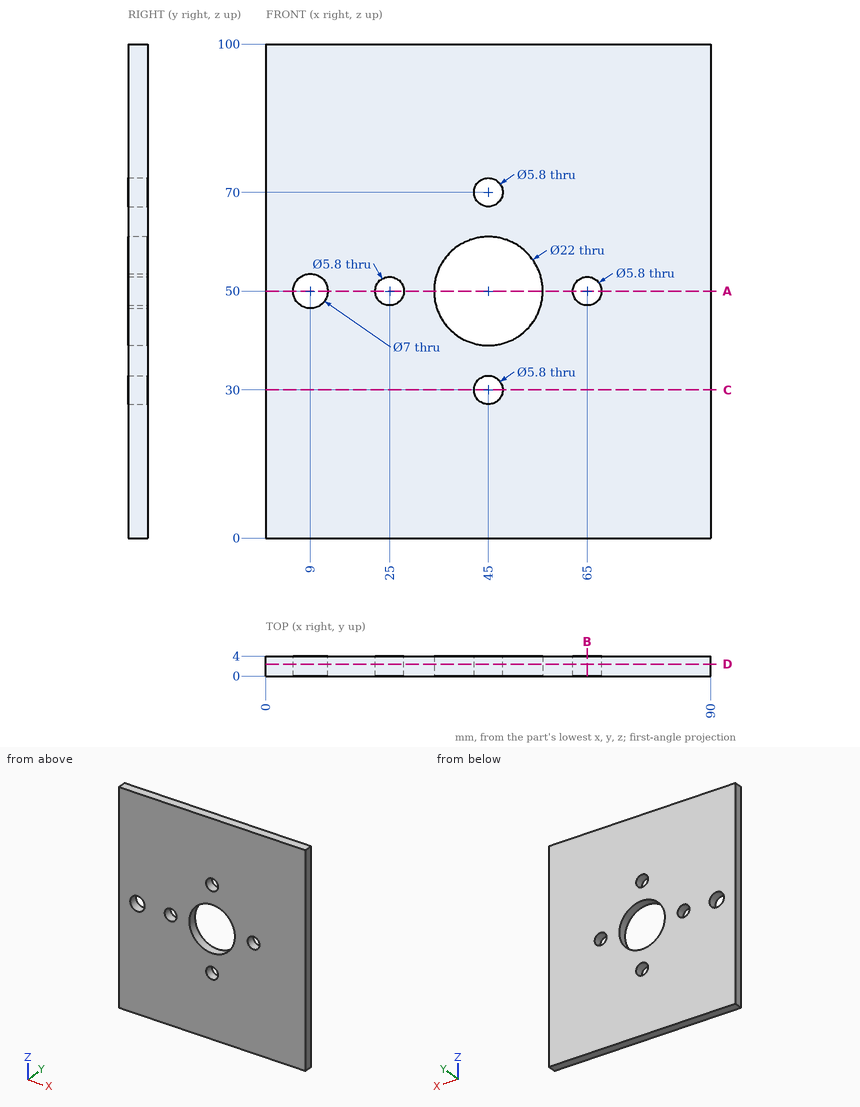
Check sheet for the drawn part. Datum: minimum x, y, z corner. Units: mm. Round coordinates to 2 decimals unless told otherwise and drop trailing zeros. Write each loop counter-clockwise with the first axis right and the second up, starting at its lowest first coordinate (ties: lowest second). Pieces come first, ordered by that corner, then holes. Notation, with made-up numbers: (2, 86) -> (8, 86) arc R28 ccw to (8, 114) -> close; hole circle Ø1 at (28.5, 66.5). An arc over 180 degrees is marked (long way). Write each question's results on one line, items separated by ' | '. Start each with the question number.
1. Cross-section at A-A (z = 50). Enter the section's corners in (x, y), then the cut area to 3 significant figures.
2. Material ranges on probe 1 along X at (y, z) = (2, 50); probe 2 along Z at (x, y) = (9, 1.5); probe 3 along Z at (x, y) = (65, 2.4), recorded low to high. Write a range as from..to.
3. Cross-section at D-D (y = 2.4). Enter the section's corners in (x, z), then the cut area to 3 significant figures.
4. Cross-section at B-B (x = 65). Enter the section's corners in (y, z), then the cut area to 3 significant figures.
5. Depth check by flat-ended pin: P1, Ø13, axis at x = 45, z = 50, coming from the +Y side. Enter the tip coordinate at first touch or a pass-through.
6. Cross-section at C-C (z = 30). Enter the section's corners in (x, y), then the cut area to 3 significant figures.
Solutions:
1) outline: (0, 0) -> (5.5, 0) -> (5.5, 4) -> (0, 4) -> close; (12.5, 0) -> (22.1, 0) -> (22.1, 4) -> (12.5, 4) -> close; (27.9, 0) -> (34, 0) -> (34, 4) -> (27.9, 4) -> close; (56, 0) -> (62.1, 0) -> (62.1, 4) -> (56, 4) -> close; (67.9, 0) -> (90, 0) -> (90, 4) -> (67.9, 4) -> close | area: 198 mm2
2) probe 1: x = 0..5.5, 12.5..22.1, 27.9..34, 56..62.1, 67.9..90 | probe 2: z = 0..46.5, 53.5..100 | probe 3: z = 0..47.1, 52.9..100
3) outline: (0, 0) -> (90, 0) -> (90, 100) -> (0, 100) -> close; hole circle Ø7 at (9, 50); hole circle Ø5.8 at (25, 50); hole circle Ø22 at (45, 50); hole circle Ø5.8 at (45, 30); hole circle Ø5.8 at (45, 70); hole circle Ø5.8 at (65, 50) | area: 8,480 mm2
4) outline: (0, 0) -> (4, 0) -> (4, 47.1) -> (0, 47.1) -> close; (0, 52.9) -> (4, 52.9) -> (4, 100) -> (0, 100) -> close | area: 377 mm2
5) P1: passes through
6) outline: (0, 0) -> (42.1, 0) -> (42.1, 4) -> (0, 4) -> close; (47.9, 0) -> (90, 0) -> (90, 4) -> (47.9, 4) -> close | area: 337 mm2
